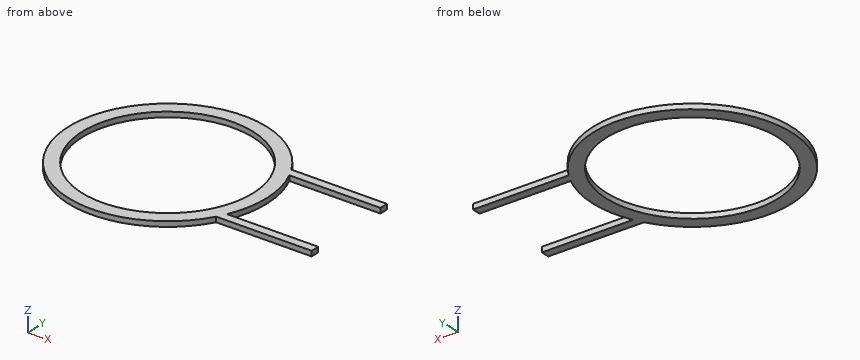
from build123d import *

# Parameters (mm, degrees)
EXTRUDE_1_DEPTH     = 3
SKETCH_5_R          = 50
CUT_EXTRUDE_1_DEPTH = 3


with BuildPart() as part:
    # 草圖1 → 填料-伸長1 (new body)
    with BuildSketch(Plane.XY):
        with BuildLine():
            Line((106, 24), (52.80151513, 24))
            ThreePointArc((52.80151513, 24), (58, 0), (52.80151513, -24))
            Line((52.80151513, -24), (106, -24))
            Line((106, -24), (106, -29))
            Line((106, -29), (50.229473419, -29))
            ThreePointArc((50.229473419, -29), (-58, 0), (50.229473419, 29))
            Line((50.229473419, 29), (106, 29))
            Line((106, 29), (106, 24))
        make_face()
    extrude(amount=EXTRUDE_1_DEPTH)

    # 草圖5 → 除料-伸長1 (cut)
    with BuildSketch(Plane.XY.offset(3)):
        Circle(SKETCH_5_R)
    extrude(amount=-CUT_EXTRUDE_1_DEPTH, mode=Mode.SUBTRACT)


solid = part.part
Verification items for the finished model (mm, model axes). Coordinates: 2 decimals unless noted, no trailing zeros. Order: outer loops, then holes, each group sorted by start corner. A loop starts at its lowest first (then second) coordinate and runs counter-clockwise, first axis right, second up.
Item 1: Section check B-B, the plane y = 0. Enter the section's corners in (x, z).
Filled in:
outline: (-58, 0) - (-50, 0) - (-50, 3) - (-58, 3) - close; (50, 0) - (58, 0) - (58, 3) - (50, 3) - close
Item 2: Section check C-C, the plane z = 1.9. Enter the section's corners in (x, y), then the cut area to 3 significant figures.
Filled in:
outline: (50.23, -29) - (106, -29) - (106, -24) - (52.8, -24) arc R58 ccw to (52.8, 24) - (106, 24) - (106, 29) - (50.23, 29) arc R58 ccw (long way) to start; hole circle Ø100 at (0, 0)
area: 3,260 mm2
Item 3: Section check A-A, the plane x = 90.5. Enter the section's corners in (y, z), then the cut area to 3 significant figures.
Filled in:
outline: (-29, 0) - (-24, 0) - (-24, 3) - (-29, 3) - close; (24, 0) - (29, 0) - (29, 3) - (24, 3) - close
area: 30.0 mm2
Item 4: Depth check by flat-ended pin: pin 1 (0.9 mm diameter, centred on x = 85.5, z = 1.5, fed in from +Y); pin 2 (1.5 mm diameter, centred on y = -0.5, z = 2.5, fed in from -X); pin 3 (1.5 mm diameter, centred on x = 83, z = 1, fed in from -Y); pin 4 (12 mm diameter, centred on x = 71.5, y = -36, fed in from -Z). Enter the tip coordinate at first touch or a pass-through.
Filled in:
pin 1: stops at y = 29
pin 2: stops at x = -58
pin 3: stops at y = -29
pin 4: passes through
Item 5: Material ranges on L1, parallel to Y at x = 0, z = 0.9; L2, parallel to X at y = -40, z = 2.65; L3, parallel to X at y = -2, z = 1.35, recorded low to high.
Filled in:
L1: y = -58 to -50, 50 to 58
L2: x = -42 to -30, 30 to 42
L3: x = -57.97 to -49.96, 49.96 to 57.97
